Part model, mm, in its own coordinate system. A direction names the side the tool comes from. Round coordinates to 2 decimals unless told otherwise and drop trailing zeros. Write each loop counter-clockwise with the first axis right and the second up, starting at its lowest first coordinate (ties: lowest second). Pieces come first, ordered by that corner, then holes. Notation, with made-up numbers: M 29.5,70.5 L 81.5,70.5 A22 cw 81.5,82.5 Z; hole C -5,18 d3. An arc over 180 degrees is marked long. Answer as a JSON object with one key per item and string values. Group by question number.
1. Two-plate mould, pull along Y, no slides. Class faces 1 (the face through (0, 0, 0)), 2 (the face through (21.84, 3.1, 0.69)), 3 (the face through (9.651, -2.581, -11.623)): +Y half, -Y half, draft (parallel to the pull), parting line (faces both ways), or undercut.
2. Band-saw the part on A-A, the plane x = 28. Write the cut outline in (y, z) (3 decimals).
3. Band-saw the part on C-C, the plane x = 16. Write the cut outline in (y, z) (3 decimals), plus the area to 3 significant figures.
4. Drop flat-ended pins along their axis: pin 1 (5.5 mm diameter, centred on y = 0, z = 0, fed in from +X); pin 2 (6 mm diameter, centred on x = 4, y = -8, fed in from -Z); pin 3 (3 mm diameter, centred on x = 21, y = 5.5, fed in from +Z). Give the stop position or say it passes through.
5. Which spindle directions (+Z, -Z, +X, -X, +Y, -Y) get a long thin tool onto all of the face, cutting with end or side? Do faces 4 (the face through (25.482, -7.559, -5.796)), 5 (the face through (31.75, 4, 0)). Say none if no direction does.
6. Drill centre lines: line 1 (Y direction, x = 26.5, z = 0) (3 decimals); line 2 (Y direction, x = 18, z = 0) (3 decimals). Where is each one in solid material? Low to high. Write a range as from..to.
7. Band-saw the part on B-B, the plane x = 5.5. Write the cut outline in (y, z).
Autodesk Fusion 360 part; units mm, degrees
sketch "Sketch1" plane through (0, 0, 0) normal (0, 0, 1) x (1, 0, 0)
  line L0 (0, 0) -> (0, 11.9062)
  line L1 (0, 11.9062) -> (19.05, 11.9063)
  line L2 (19.05, 11.9063) -> (19.05, 9.525)
  line L3 (19.05, 9.525) -> (31.75, 9.525)
  line L4 (31.75, 9.525) -> (31.75, 0)
  line L5 (31.75, 0) -> (0, 0)
  dimension "d1" = 11.9062
  dimension "d2" = 9.525
  dimension "d3" = 12.7
  dimension "d4" = 19.05
revolve "Revolve1" add sketch "Sketch1" angle 360 about axis through (31.75, 0, 0) along (-1, 0, 0)
hole "Hole1" at (31.75, 0, 0) direction (-1, 0, 0) diameter 6.35 depth 19.05 tip angle 118
chamfer "Chamfer1" distance 0.508 angle 45 5 edges at (0, -4.3055, 11.1005) (19.05, -4.3055, 11.1005) (19.05, -3.4444, 8.8804) (31.75, -3.4444, 8.8804) (31.75, -2.9601, 1.1481)
equation "d1 = ( 15 / 32 ) * 1 in"
Worked answers:
{
 "1": {"face 1": "draft", "face 2": "undercut", "face 3": "parting line"},
 "2": {"outline": "C 0,0 d19.05; hole C 0,0 d6.35"},
 "3": {"outline": "C 0,0 d23.812; hole C 0,0 d6.35", "area": "414 mm^2"},
 "4": {"pin 1": "stops at x = 12.44", "pin 2": "stops at z = -10.81", "pin 3": "stops at z = 8.64"},
 "5": {"face 4": "+X", "face 5": "+Z, -Z, +X, +Y, -Y"},
 "6": {"line 1": "y = -9.525..-3.175, 3.175..9.525", "line 2": "y = -11.906..-3.175, 3.175..11.906"},
 "7": {"outline": "C 0,0 d23.81"}
}
